```python
from build123d import *

# Parameters (mm, degrees)
F1_DEPTH = 914.4
F2_T     = -3.175
F3_W     = 753.724518
F3_H     = 3.175
F4_DEPTH = 304.8
F5_R     = 50.8


with BuildPart() as f1:
    # F0 (on Top) → F1 (new body)
    with BuildSketch(Plane.XY):
        Polygon((278.911358, -381), (381, 0), (-381, 0), (-278.911358, -381), align=None)
    extrude(amount=F1_DEPTH)

    # F2
    f2_openings = [f1.faces().sort_by_distance(p)[0] for p in [
        (0, -180.676516, 914.4),
    ]]
    offset(amount=F2_T, openings=f2_openings)

    # F3 (on face) → F4 (join)
    with BuildSketch(Plane.XY.offset(914.4)):
        with Locations((0, -1.5875)):
            Rectangle(F3_W, F3_H)
    extrude(amount=F4_DEPTH)

    # F5
    f5_edges = [f1.edges().sort_by_distance(p)[0] for p in [
        (376.862259, -1.5875, 1219.2),
        (-376.862259, -1.5875, 1219.2),
    ]]
    fillet(f5_edges, radius=F5_R)


solid = f1.part
```
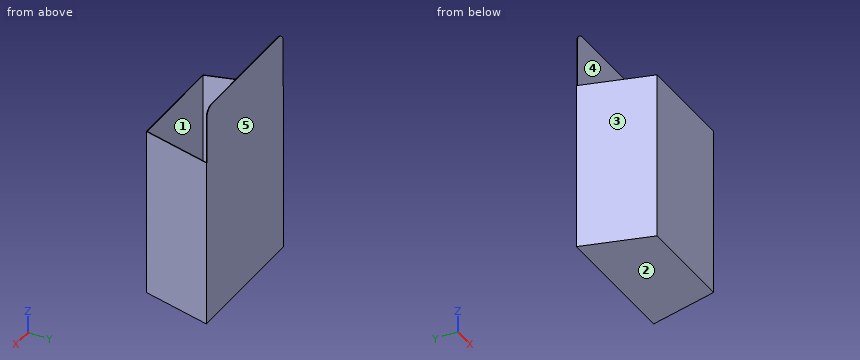
For this review, take the finished solid that the model builds, in its own axes (mm). Face numbers are marked on the shaded views. A direction names the side the tool comes from. Give positions to 0.01 mm unless a question says otherwise; leave off trailing zeros. Loops run counter-clockwise (first coordinate to the right, second up) from the corner with the lowest first, then second, coordinate; pieces in that order, holes last. Notation, with made-up numbers: M 34.25,18 L 63.25,18 A12 cw 63.25,22 Z; hole C 35,-29.5 d5. An arc over 180 degrees is marked long. One line per item, written item: value. Start each with the question number.
Q1. Draft analysis for pull direction X (two halves, no side actions). For the marked faces 3, 4 and 5, state which applies: released by +X, released by -X, zero draft, split by the parting line, or undercut.
Q2. Clearance check with flat-ended pins moving along their axes: pin 1 Ø1 at (y, z) = (-1, 1082) entering from +X; pin 2 Ø2 at (y, z) = (-320.5, 437) entering from -X; pin 3 Ø1 at (y, z) = (-1.5, 1028) entering from -X. State where each tip first meets the part, or that it passes through.
Q3. Add section A-A (x = 234). Give the boundary of the cut face in (y, z) (3 decimals), and give its area (3 significant figures).
Q4. Add section C-C (y = -275). Give the boundary of the cut face in (x, z) (3 decimals), and give its area (3 significant figures).
Q5. Machinability: for the marked faces 1 and 2, which of the approach directions +Z, -Z, +X, -X, +Y, -Y give a long, thin tool a straight path to every point of the face, cutting with its end or side? Answer none if there is none.
Q6. For L1, parallel to Y at x = 181, z = 188 (3 decimals); L2, parallel to Z at x = -44.5, y = -326.5 (3 decimals); L3, parallel to Y at x = -208, z = 1077.5 (3 decimals), list the stretches that pass through material, from the lowest coordinate up.
Q7. Add section B-B (z = 196.5). Give the boundary of the cut face in (x, y) (3 decimals), and give its area (3 significant figures).
Reply:
1. face 3: released by -X
1. face 4: undercut
1. face 5: zero draft
2. pin 1: x = 376.86
2. pin 2: x = -295.39
2. pin 3: x = -376.86
3. outline: M -381,0 L 0,0 L 0,1219.2 L -3.175,1219.2 L -3.175,3.175 L -377.825,3.175 L -377.825,914.4 L -381,914.4 Z
3. area: 7,960 mm²
4. outline: M -307.314,0 L 307.314,0 L 307.314,914.4 L 304.027,914.4 L 304.027,3.175 L -304.027,3.175 L -304.027,914.4 L -307.314,914.4 Z
4. area: 7,940 mm²
5. face 1: +Z
5. face 2: -Z, +X, -X, +Y, -Y
6. L1: -381 to -377.825, -3.175 to 0
6. L2: 0 to 3.175
6. L3: -3.175 to 0
7. outline: M -381,0 L -278.911,-381 L 278.911,-381 L 381,0 Z; hole M -376.862,-3.175 L -276.475,-377.825 L 276.475,-377.825 L 376.862,-3.175 Z
7. area: 6,650 mm²
